```python
from build123d import *

# Parameters (mm, degrees)
F0_R     = 2.2479
F1_DEPTH = 5.08


with BuildPart() as f1:
    # F0 (on Top) → F1 (new body)
    with BuildSketch(Plane.XY):
        Polygon((0, 31.75), (0, 38.1), (-27.496307, 15.875), (-32.995568, 19.05), (-27.496307, -15.875), (-32.995568, -19.05), (0, -31.75), (0, -38.1), (27.496307, -15.875), (32.995568, -19.05), (27.496307, 15.875), (32.995568, 19.05), align=None)
        with Locations((-20.897193, -12.065)):
            Circle(F0_R, mode=Mode.SUBTRACT)
        with Locations((0, -24.13)):
            Circle(F0_R, mode=Mode.SUBTRACT)
        with Locations((20.897193, -12.065)):
            Circle(F0_R, mode=Mode.SUBTRACT)
        with Locations((-20.897193, 12.065)):
            Circle(F0_R, mode=Mode.SUBTRACT)
        Polygon((-7.332348, 0), (-3.666174, 6.35), (3.666174, 6.35), (7.332348, 0), (3.666174, -6.35), (-3.666174, -6.35), align=None, mode=Mode.SUBTRACT)
        with Locations((20.897193, 12.065)):
            Circle(F0_R, mode=Mode.SUBTRACT)
        with Locations((0, 24.13)):
            Circle(F0_R, mode=Mode.SUBTRACT)
    extrude(amount=F1_DEPTH)


solid = f1.part
```
CAD build for the part. Positions are in the model's coordinates, mm. A direction names the side the tool comes from. Coordinates: 2 decimals unless noted, no trailing zeros. Write each loop counter-clockwise with the first axis right and the second up, starting at its lowest first coordinate (ties: lowest second). Pieces come first, ordered by that corner, then holes.
(1) Cut at D-D, the plane x = -21. List the corners of the cut face in (y, z), and give its area (3 significant figures).
(2) Two-plate mould, pull along Y, no slides. Class faces 4 (the face through (0, 9, 0)), 5 (the face through (-13.56, 27.14, 2.5)), 6 (the face through (30.21, -17.44, 2.5)), 7 (the face through (5.474, 3.219, 2.504)): +Y half, -Y half, draft (parallel to the pull), parting line (faces both ways), or undercut.
(3) Cut at C-C, the plane z = 4. List the corners of the cut face in (x, y) (3 decimals).
(4) Drill centre lines: probe 1 along Y at (x, z) = (22, 0.85); probe 2 along Y at (x, z) = (21.5, 4.1); probe 3 along X at (y, z) = (1.5, 0.55). Where is each one in solid material? Low to high.
(5) Cut at A-A, the plane x = 29. List the corners of the cut face in (y, z), and give its area (3 significant figures).
(6) Cut at B-B, the plane y = -3.5. List the corners of the cut face in (x, z).
(7) Flat gauge pins, fed straight in: pin 1 (1.5 mm diameter, centred on y = -33.5, z = 3.5, fed in from -X); pin 2 (2.5 mm diameter, centred on x = 0, z = 3, fed in from +Y); pin 3 (1 mm diameter, centred on x = -17.5, z = 2.5, fed in from -Y). Where does each tip first touch, or does it go through?
(8) 3-axis set-ups, long thin cutter, end or side, ignore diameter. For faces 1 (the face through (0, -35, 3)), 2 (the face through (0, -6.35, 3)), 3 (the face through (0, 35, 3)): which of +Z, -Z, +X, -X, +Y, -Y reach the whole face in a straight line?
Geometry says:
1. outline: (-23.67, 0) - (-14.31, 0) - (-14.31, 5.08) - (-23.67, 5.08) - close; (-9.82, 0) - (9.82, 0) - (9.82, 5.08) - (-9.82, 5.08) - close; (14.31, 0) - (21.13, 0) - (21.13, 5.08) - (14.31, 5.08) - close
1. area: 182 mm2
2. face 4: draft
2. face 5: +Y half
2. face 6: -Y half
2. face 7: undercut
3. outline: (-32.996, -19.05) - (0, -31.75) - (0, -38.1) - (27.496, -15.875) - (32.996, -19.05) - (27.496, 15.875) - (32.996, 19.05) - (0, 31.75) - (0, 38.1) - (-27.496, 15.875) - (-32.996, 19.05) - (-27.496, -15.875) - close; hole circle Ø4.496 at (-20.897, -12.065); hole circle Ø4.496 at (-20.897, 12.065); hole (-7.332, 0) - (-3.666, -6.35) - (3.666, -6.35) - (7.332, 0) - (3.666, 6.35) - (-3.666, 6.35) - close; hole circle Ø4.496 at (0, -24.13); hole circle Ø4.496 at (0, 24.13); hole circle Ø4.496 at (20.897, -12.065); hole circle Ø4.496 at (20.897, 12.065)
4. probe 1: y = -20.32 to -14.02, -10.11 to 10.11, 14.02 to 23.28
4. probe 2: y = -20.72 to -14.23, -9.9 to 9.9, 14.23 to 23.47
4. probe 3: x = -30.23 to -6.47, 6.47 to 29.76
5. outline: (-16.74, 0) - (6.33, 0) - (6.33, 5.08) - (-16.74, 5.08) - close; (16.74, 0) - (20.59, 0) - (20.59, 5.08) - (16.74, 5.08) - close
5. area: 137 mm2
6. outline: (-29.44, 0) - (-5.31, 0) - (-5.31, 5.08) - (-29.44, 5.08) - close; (5.31, 0) - (30.55, 0) - (30.55, 5.08) - (5.31, 5.08) - close
7. pin 1: stops at x = 0
7. pin 2: stops at y = 38.1
7. pin 3: stops at y = -25.21
8. face 1: +Z, -Z, -X, -Y
8. face 2: +Z, -Z
8. face 3: +Z, -Z, +X, +Y
